Autodesk Inventor part; units mm, degrees
ref_plane "YZ Plane" through (0, 0, 0) normal (1, 0, 0) x (0, 1, 0)
ref_plane "XZ Plane" through (0, 0, 0) normal (0, 1, 0) x (-1, 0, 0)
ref_plane "XY Plane" through (0, 0, 0) normal (0, 0, 1) x (1, 0, 0)
sketch "Sketch1" plane through (0, 0, 0) normal (0, 0, 1) x (1, 0, 0)
  line L0 (0, 0) -> (114.3, 0)
  line L1 (114.3, 0) -> (114.3, 44.45)
  line L2 (114.3, 44.45) -> (0, 44.45)
  line L3 (0, 44.45) -> (0, 0)
  dimension "d0" = 114.3
  dimension "d1" = 44.45
extrude "Extrusion1" add sketch "Sketch1" along normal blind 44.45
sketch "Sketch2" plane through (114.3, 0, 0) normal (1, 0, 0) x (0, 0, -1)
  line L0 (0, 44.45) -> (-44.45, 44.45)
  line L1 (-25.4, 44.45) -> (-19.05, 44.45)
  line L2 (-19.05, 44.45) -> (-19.05, 38.1)
  line L3 (-19.05, 38.1) -> (-25.4, 38.1)
  line L4 (-25.4, 38.1) -> (-25.4, 44.45)
  line L5 (-44.45, 0) -> (-44.45, 44.45)
  line L6 (0, 0) -> (0, 44.45)
  dimension "d4" = 19.05
  dimension "d5" = 19.05
  dimension "d6" = 6.35
  dimension "d7" = 6.35
extrude "Extrusion2" add sketch "Sketch2" along normal blind 12.7
properties part number "batery" material "Rubber"
Design review of the part built by this model. Coordinates are the model's own, in mm. A direction names the side the tool comes from. Give positions to 0.01 mm unless a question says otherwise; leave off trailing zeros. Loops run counter-clockwise (first coordinate to the right, second up) from the corner with the lowest first, then second, coordinate; pieces in that order, holes last. Notation, with made-up numbers: M -7,-9.75 L 19,-9.75 A26 ccw 19,4.25 Z; hole C 51,88.25 d5. An arc over 180 degrees is marked long. Return JSON: item names as keys, results as strings. Group by question number.
Item 1: We need section C-C (z = 23). Give the boundary of the cut face in (x, y), and give its area (3 significant figures).
Item 2: Tool access review of faces 1 (the flat face through (121, 38.1, 22)), 2 (the flat face through (121, 41, 25.4)), 3 (the flat face through (121, 41, 19.05)): name each direction out of +Z, -Z, +X, -X, +Y, -Y from which nothing blocks a thin tool from reaching the whole face with its end or side.
Item 3: We need section A-A (z = 36). Give the boundary of the cut face in (x, y), and give its area (3 significant figures).
Item 4: Insertion check: pin 1 Ø1 at (x, z) = (60.5, 27) entering from -Y; pin 2 Ø8 at (y, z) = (29.5, 38) entering from +X; pin 3 Ø5 at (x, z) = (120, 22.5) entering from -Y; pin 4 Ø3 at (x, y) = (120.5, 41.5) entering from +Z. Each pin has a flat end and moves straight along its axis. Give the tip position at first contact, or say it passes through.
Item 5: For probe 1 along X at (y, z) = (36, 27.5), list the stretches that pass through material, from the lowest coordinate up.
Output:
{
 "1": {"outline": "M 0,0 L 114.3,0 L 114.3,38.1 L 127,38.1 L 127,44.45 L 0,44.45 Z", "area": "5,160 mm^2"},
 "2": {"face 1": "+Z, -Z, +X, -Y", "face 2": "+Z, +X, +Y, -Y", "face 3": "-Z, +X, +Y, -Y"},
 "3": {"outline": "M 0,0 L 114.3,0 L 114.3,44.45 L 0,44.45 Z", "area": "5,080 mm^2"},
 "4": {"pin 1": "stops at y = 0", "pin 2": "stops at x = 114.3", "pin 3": "stops at y = 38.1", "pin 4": "stops at z = 25.4"},
 "5": {"probe 1": "x = 0 to 114.3"}
}
